Read the model definition and answer for the solid it produces. Units are mm, in the model's axes. A direction names the side the tool comes from. Coordinates: 2 decimals unless noted, no trailing zeros. Write each loop counter-clockwise with the first axis right and the second up, starting at its lowest first coordinate (ties: lowest second). Pieces come first, ordered by that corner, then holes. Notation, with made-up numbers: (17.25, -20.5) -> (30.25, -20.5) arc R17 cw to (30.25, -2.5) -> close; hole circle Ø10 at (51.5, -22). An arc over 180 degrees is marked (long way). One line per item, written item: value. Start each with the question number.
1. Consider line 1 along Y through (x, z) = (-8, 3.25); line 2 along Y through (x, z) = (87, 2); line 3 along Y through (x, z) = (114, 2.5). Determine where each line is inside the solid, lowest interval first.
2. Find section A-A, the plane z = 1.75. Write down the section's boundary in (x, y).
3. Find section C-C, the plane x = 21. Write down the section's boundary in (y, z), and give its area (3 significant figures).
4. Given P1, Ø3, axis at y = -158, z = 1.5, coming from the -X side; P2, Ø1.9, axis at y = 165.5, z = 3.5, coming from the -X side; P3, Ø3, axis at y = -111.5, z = 5, coming from the -X side, each flat-ended and moving along its own axis, determine where each tip first touches the part or whether it passes through.
5. Find section B-B, the plane x = 49. Write down the section's boundary in (y, z).
6. Find section D-D, the plane x = 90.5. Write down the section's boundary in (y, z).
7. For faces 4 (the flat face through (-10, 161.152, 3)), 5 (the flat face through (163.83, -63, 3)), 6 (the flat face through (160, -76.2, 3)), 7 (the flat face through (16, -161.29, 3)), determine the directions among +Z, -Z, +X, -X, +Y, -Y from which every point of the face is accessible in a straight line to the end or side of a thin tool.
8. For a pull along X with two mould halves and no side action, classify faces 1 (the flat face through (159, -68.262, 3)), 2 (the flat face through (150, -12, 6.35)), 3 (the flat face through (6.348, -165, 3)) as pulls with the +X half, pulls with the -X half, needs draft (parallel to the pull), parting line crosses it, or undercut.
Autodesk Inventor part; units mm, degrees
ref_plane "YZ Plane" through (0, 0, 0) normal (1, 0, 0) x (0, 1, 0)
ref_plane "XZ Plane" through (0, 0, 0) normal (0, 1, 0) x (-1, 0, 0)
ref_plane "XY Plane" through (0, 0, 0) normal (0, 0, 1) x (1, 0, 0)
sketch "Sketch1" plane through (0, 0, 0) normal (0, 0, 1) x (1, 0, 0)
  arc A0 (6.3485, -145.912) -> (6.35, 145.9119) centre (0, 0) ccw
  line L0 (6.35, -150.9919) -> (6.35, -151.13)
  line L1 (6.35, 145.9119) -> (6.35, 168.7906)
  line L2 (0, 0) -> (0, 200.5264) construction
  line L3 (6.35, 145.9119) -> (6.35, 150.9919) construction
  line L4 (6.35, 150.9919) -> (-25.4, 150.9919)
  line L5 (-25.4, 150.9919) -> (-25.4, 161.1519)
  line L6 (-25.4, 161.1519) -> (6.35, 161.1519)
  line L7 (0, -146.05) -> (0, 0) construction
  line L8 (168.91, 0) -> (168.91, -76.2)
  line L9 (168.91, -76.2) -> (150.7453, -76.2)
  line L10 (0, 0) -> (0, -63.5) construction
  line L11 (0, -63.5) -> (158.75, -63.5) construction
  line L12 (158.75, -58.7375) -> (163.83, -58.7375)
  line L13 (163.83, -58.7375) -> (163.83, -68.2625)
  line L14 (163.83, -68.2625) -> (153.67, -68.2625)
  line L15 (153.67, -68.2625) -> (153.67, -58.7375)
  line L16 (153.67, -58.7375) -> (158.75, -58.7375)
  arc A1 (6.3485, -168.7907) -> (150.7453, -76.2) centre (0, 0) ccw
  line L17 (6.35, 161.1519) -> (-6.35, 161.1519) construction
  line L18 (-6.35, 161.1519) -> (-6.35, 168.7906) construction
  line L19 (0, -146.05) -> (0, -151.13) construction
  line L20 (6.3485, -151.13) -> (25.4, -151.13)
  line L21 (25.4, -151.13) -> (25.4, -161.29)
  line L22 (25.4, -161.29) -> (6.3485, -161.29)
  arc A2 (168.91, 0) -> (6.35, 168.7906) centre (0, 0) ccw
  line L23 (0, -146.05) -> (6.3485, -145.912) construction
  line L24 (6.3485, -145.912) -> (6.3485, -151.13)
  line L25 (6.3485, -161.29) -> (6.3485, -168.7907)
  line L26 (6.3485, -145.912) -> (6.3485, -151.13) construction
  line L27 (6.3485, -161.29) -> (6.3485, -184.4747) construction
  point P0 (6.35, -145.9119)
  point P1 (0.0447, 168.91)
  point P2 (6.3947, 145.9099)
  dimension "d51" = 292.1
  dimension "d72" = 6.35
  dimension "d73" = 5.08
  dimension "d75" = 31.75
  dimension "d76" = 10.16
  dimension "d82" = 76.2
  dimension "d86" = 63.5
  dimension "d87" = 158.75
  dimension "d89" = 4.7625
  dimension "d90" = 5.08
  dimension "d91" = 9.525
  dimension "d92" = 10.16
  dimension "d93" = 4.7625
  dimension "d100" = 12.7
  dimension "d101" = 5.08
  dimension "d103" = 25.4
  dimension "d104" = 10.16
  dimension "d105" = 6.35
  dimension "d106" = 7.5007
  dimension "d107" = 25.4
extrude "Extrusion18" add sketch "Sketch1" along normal blind 6.35
properties part number "TopmaleHoopSection_v2"
Answer block:
1. line 1: y = 150.99 to 161.15
1. line 2: y = -144.78 to -117.31, 117.31 to 144.78
1. line 3: y = -124.64 to -91.29, 91.29 to 124.64
2. outline: (-25.4, 150.99) -> (6.35, 150.99) -> (6.35, 145.91) arc R146.05 cw to (6.35, -145.91) -> (6.35, -150.99) -> (6.35, -151.13) -> (25.4, -151.13) -> (25.4, -161.29) -> (6.35, -161.29) -> (6.35, -168.79) arc R168.91 ccw to (150.75, -76.2) -> (168.91, -76.2) -> (168.91, 0) arc R168.91 ccw to (6.35, 168.79) -> (6.35, 161.15) -> (-25.4, 161.15) -> close; hole (153.67, -68.26) -> (163.83, -68.26) -> (163.83, -58.74) -> (153.67, -58.74) -> close
3. outline: (-167.6, 0) -> (-161.29, 0) -> (-161.29, 6.35) -> (-167.6, 6.35) -> close; (-151.13, 0) -> (-144.53, 0) -> (-144.53, 6.35) -> (-151.13, 6.35) -> close; (144.53, 0) -> (167.6, 0) -> (167.6, 6.35) -> (144.53, 6.35) -> close
3. area: 228 mm2
4. P1: stops at x = 25.4
4. P2: stops at x = 6.35
4. P3: stops at x = 92.53
5. outline: (-161.65, 0) -> (-137.58, 0) -> (-137.58, 6.35) -> (-161.65, 6.35) -> close; (137.58, 0) -> (161.65, 0) -> (161.65, 6.35) -> (137.58, 6.35) -> close
6. outline: (-142.62, 0) -> (-114.63, 0) -> (-114.63, 6.35) -> (-142.62, 6.35) -> close; (114.63, 0) -> (142.62, 0) -> (142.62, 6.35) -> (114.63, 6.35) -> close
7. face 4: +Z, -Z, -X, +Y
7. face 5: +Z, -Z
7. face 6: +Z, -Z, +X, -Y
7. face 7: +Z, -Z, -X
8. face 1: undercut
8. face 2: needs draft
8. face 3: pulls with the -X half
